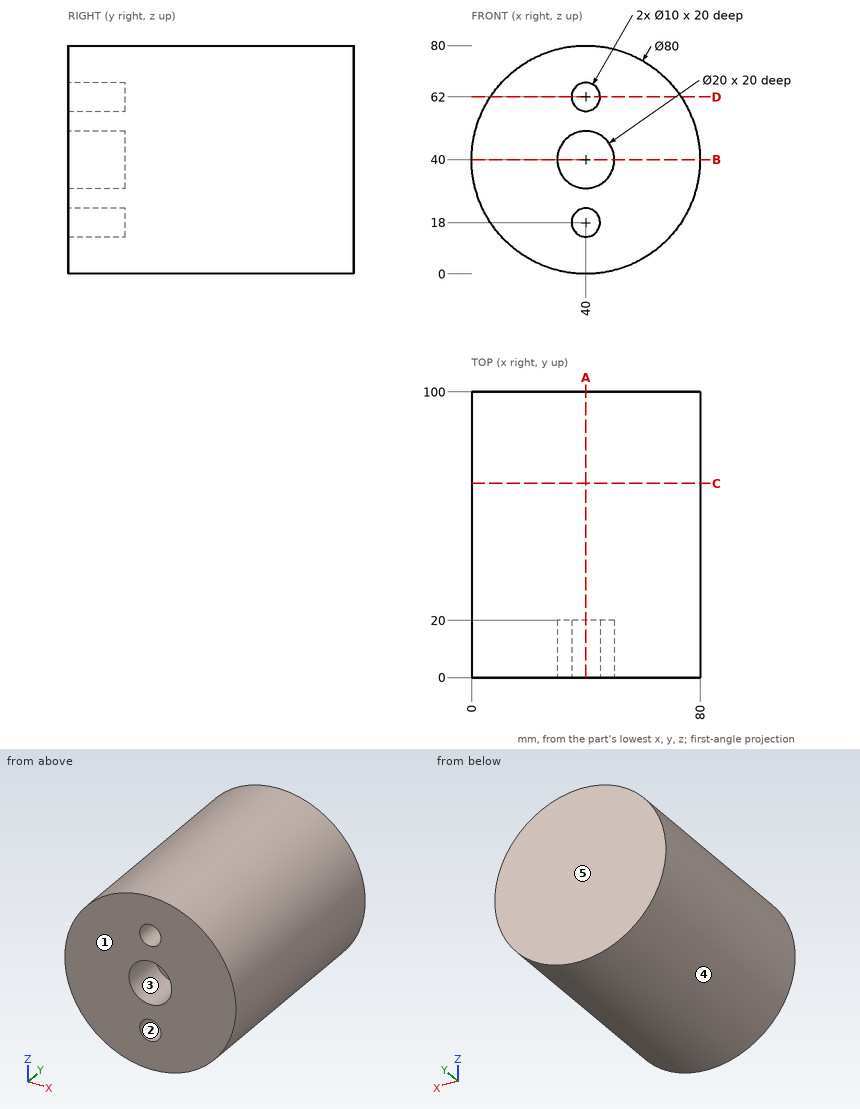
Can you work these out from the drawing? Everything is in mm from the part's minimum corner. A direction names the side the tool comes from. Coordinates: 2 decimals unless noted, no trailing zeros. Loops run counter-clockwise (first coordinate to the right, second up) from the corner with the lowest first, then second, coordinate; pieces in that order, holes last. Notation, with made-up numbers: M -17.5,24 L 25.5,24 A24 ccw 25.5,34 Z; hole C -32,44 d10. An arc over 180 degrees is marked long. Put each result on its own line as item: value. Start each with the question number.
(1) Suppose I cut it at C-C on y = 68. Please give me the cut outline in (x, z).
(2) I need wall thicknesses on line 1 (X direction, y = 8, z = 40); line 2 (Y direction, x = 38.5, z = 34); line 3 (Z direction, x = 43, y = 4). Which ranges of each line are inside material? Lowest first, please. Write a range as from..to.
(3) Will these pins go through, and if not, where does the flat tip stop? P1, Ø1, axis at y = 14, z = 37, coming from the -X side; P2, Ø3, axis at x = 65.5, y = 62.5, coming from the +Z side; P3, Ø5, axis at x = 22.5, y = 69.5, coming from the -Z side.
(4) Thinking about a two-plate mould opening in Z: for the marked faces 3, 4 and 5, which applies, pulls with the +Z half, pulls with the -Z half, needs draft (parallel to the pull), parting line crosses it, or undercut?
(5) Suppose I cut it at A-A on x = 40. Please give me the cut outline in (y, z), then the cut area to 3 significant figures.
(6) For the marked faces 1 and 2, which set-ups out of +Z, -Z, +X, -X, +Y, -Y let a thin tool reach every point of the face, with its end or its side?
(7) Suppose I cut it at D-D on z = 62. Please give me the cut outline in (x, y).
(8) Suppose I cut it at B-B on z = 40. Please give me the cut outline in (x, y), then the cut area to 3 significant figures.
Solutions:
1. outline: C 40,40 d80
2. line 1: x = 0..30, 50..80
2. line 2: y = 20..100
2. line 3: z = 0.11..14, 22..30.46, 49.54..58, 66..79.89
3. P1: stops at x = 0.08
3. P2: stops at z = 72
3. P3: stops at z = 2.92
4. face 3: undercut
4. face 4: parting line crosses it
4. face 5: needs draft
5. outline: M 0,0 L 100,0 L 100,80 L 0,80 L 0,67 L 20,67 L 20,57 L 0,57 L 0,50 L 20,50 L 20,30 L 0,30 L 0,23 L 20,23 L 20,13 L 0,13 Z
5. area: 7,200 mm2
6. face 1: +Z, -Z, +X, -X, -Y
6. face 2: -Y
7. outline: M 6.59,0 L 35,0 L 35,20 L 45,20 L 45,0 L 73.41,0 L 73.41,100 L 6.59,100 Z
8. outline: M 0,0 L 30,0 L 30,20 L 50,20 L 50,0 L 80,0 L 80,100 L 0,100 Z
8. area: 7,600 mm2
